Here's how the part is built. I have some questions about the finished solid (model axes, mm). A direction names the side the tool comes from. Coordinates: 2 decimals unless noted, no trailing zeros. Order: outer loops, then holes, each group sorted by start corner. A loop starts at its lowest first (then second) coordinate and runs counter-clockwise, first axis right, second up. Notation, with made-up numbers: (14, -1) - (46, -1) arc R12 cw to (46, 6) - close; hole circle Ø9 at (-23, 82.25). An arc over 180 degrees is marked (long way). Answer as CSV lines item,"result". Start each with the question number.
Q1. Thinking about a two-plate mould opening in Z: for faces 1 (the face through (1.57, 90.13, -28.6)), 2 (the face through (1.565, 94.623, 10.911)), 3 (the face through (1.57, -2.9, 3.78)), which applies, released by +Z, released by -Z, zero draft, split by the parting line, or undercut?
Q2. Suppose I cut it at A-A (z = -8). Please give me the cut outline in (x, y) (3 decimals), then the cut area to 3 significant figures.
Q3. For pin 1 Ø1 at (x, z) = (2.5, -59) entering from -Y; pin 2 Ø1.5 at (x, y) = (2, 78) entering from +Z, each with a flat end and sliding along its axis, tell me the tip position at first contact or that it passes through.
Q4. Suppose I cut it at D-D (y = 61). Please give me the cut outline in (x, z) (3 decimals), then the cut area to 3 significant figures.
Q5. I need wall thicknesses on line 1 (Y direction, x = 1.7, z = 0); line 2 (Y direction, x = 1, z = 1.5); line 3 (Y direction, x = 0.35, z = 9.5). Which ranges of each line are inside material? Lowest first, please.
Q6. Suppose I cut it at C-C (x = 0.85). Count the separate pieces of the cut face and the enclosed holes in it, then the cut area to 3 significant figures.
Q7. For faces 4 (the face through (1.565, 69.364, 8.228)), 5 (the face through (0, 39, -34)), which set-ups out of +Z, -Z, +X, -X, +Y, -Y let a thin tool reach every point of the face, with its end or its side?
from build123d import *

# Parameters (mm, degrees)
SKETCH1_R           = 4.7625
SKETCH1_R_2         = 3.175
BOSS_EXTRUDE1_DEPTH = 3.175


with BuildPart() as part:
    # Sketch1 → Boss-Extrude1 (new body)
    with BuildSketch(Plane(origin=(0, 0, 0), x_dir=(0, 0, -1), z_dir=(1, 0, 0))):
        with BuildLine():
            Line((5.788160309, -18.149371896), (68.599953325, 1.882435781))
            ThreePointArc((68.599953325, 1.882435781), (76.614344046, 9.474471101), (75.657464978, 20.472372782))
            Line((75.657464978, 20.472372782), (42.273855579, 76.621067209))
            ThreePointArc((42.273855579, 76.621067209), (28.363289988, 90.266896448), (9.525, 95.25))
            Line((9.525, 95.25), (0, 95.25))
            ThreePointArc((0, 95.25), (-11.065305521, 94.60508186), (-21.980769231, 92.679060656))
            ThreePointArc((-21.980769231, 92.679060656), (-31.407208087, 77.391083338), (-16.119230769, 67.964644481))
            ThreePointArc((-16.119230769, 67.964644481), (-8.114557382, 69.377060031), (0, 69.85))
            ThreePointArc((0, 69.85), (25.4, 44.45), (0, 19.05))
            ThreePointArc((0, 19.05), (-18.823496416, -2.928904691), (5.788160309, -18.149371896))
        make_face()
        Circle(SKETCH1_R, mode=Mode.SUBTRACT)
        with Locations((64.741179785, 13.982017045)):
            Circle(SKETCH1_R_2, mode=Mode.SUBTRACT)
    extrude(amount=BOSS_EXTRUDE1_DEPTH)


solid = part.part
Here are the results:
1,face 1,"released by -Z"
1,face 2,"released by +Z"
1,face 3,"undercut"
2,outline,"(0, -17.444) - (3.175, -17.444) - (3.175, 20.343) - (0, 20.343) - close; (0, 68.557) - (3.175, 68.557) - (3.175, 95.25) - (0, 95.25) - close"
2,area,"205 mm²"
3,pin 1,"stops at y = -1.34"
3,pin 2,"stops at z = 31.65"
4,outline,"(0, -51.561) - (3.175, -51.561) - (3.175, -19.268) - (0, -19.268) - close"
4,area,"103 mm²"
5,line 1,"y = -19.05 to -4.76, 4.76 to 19.05, 69.85 to 95.25"
5,line 2,"y = -18.99 to -4.52, 4.52 to 18.99, 69.83 to 95.24"
5,line 3,"y = -16.51 to 16.51, 69.2 to 94.78"
6,separate pieces,"1"
6,enclosed holes,"2"
6,area,"6,270 mm²"
7,face 4,"+X, -X"
7,face 5,"+Z, -Z, -X, +Y, -Y"
